```python
from build123d import *

# Parameters (mm, degrees)
SKETCH1_W           = 92
SKETCH1_H           = 80
BOSS_EXTRUDE1_DEPTH = 55
SKETCH2_W           = 78
SKETCH2_H           = 56
CUT_EXTRUDE1_DEPTH  = 50
SKETCH3_W           = 78
SKETCH3_H           = 5
CUT_EXTRUDE2_DEPTH  = 5
FILLET_TOP_R        = 3
FILLET_EDGES_R      = 3
FILLET_BOTTOM_R     = 1
FILLET4_R           = 1
CUT_EXTRUDE4_REACH  = 135.75
SKETCH5_W           = 14
SKETCH5_H           = 14


with BuildPart() as part:
    # Sketch1 → Boss-Extrude1 (new body)
    with BuildSketch(Plane(origin=(0, 0, 0), x_dir=(1, 0, 0), z_dir=(0, 1, 0))):
        with Locations((46, -40)):
            Rectangle(SKETCH1_W, SKETCH1_H)
    extrude(amount=BOSS_EXTRUDE1_DEPTH)

    # Sketch2 → Cut-Extrude1 (cut)
    with BuildSketch(Plane(origin=(0, 55, 0), x_dir=(1, 0, 0), z_dir=(0, 1, 0))):
        with Locations((46, -40)):
            Rectangle(SKETCH2_W, SKETCH2_H)
    extrude(amount=-CUT_EXTRUDE1_DEPTH, mode=Mode.SUBTRACT)

    # Sketch3 → Cut-Extrude2 (cut)
    with BuildSketch(Plane(origin=(0, 55, 0), x_dir=(1, 0, 0), z_dir=(0, 1, 0))):
        with Locations((46, -9.5)):
            Rectangle(SKETCH3_W, SKETCH3_H)
        with Locations((46, -70.5)):
            Rectangle(SKETCH3_W, SKETCH3_H)
    extrude(amount=-CUT_EXTRUDE2_DEPTH, mode=Mode.SUBTRACT)

    # Fillet_top
    fillet_top_edges = [part.edges().sort_by_distance(p)[0] for p in [
        (92, 55, 40),
        (46, 55, 0),
        (0, 55, 40),
        (46, 55, 80),
    ]]
    fillet(fillet_top_edges, radius=FILLET_TOP_R)

    # Fillet_edges
    # the kernel refuses this fillet: 3 mm, written as the material it takes off along each edge
    with BuildSketch(Plane(origin=(3, 52, 77), x_dir=(0, 0, 1), z_dir=(-1, 0, 0))) as fillet_edges_piece_1_section:
        Polygon((0, 0), (FILLET_EDGES_R, 0), (FILLET_EDGES_R, FILLET_EDGES_R), (0, FILLET_EDGES_R), align=None)
    fillet_edges_piece_1 = extrude(amount=FILLET_EDGES_R, mode=Mode.PRIVATE)
    fillet_edges_piece_1 = fillet_edges_piece_1 - Plane(origin=(3, 52, 77), x_dir=(0, -0.7071067811865475, -0.7071067811865475), z_dir=(-1, 0, 0)) * Sphere(FILLET_EDGES_R, mode=Mode.PRIVATE)
    add(fillet_edges_piece_1, mode=Mode.SUBTRACT)
    with BuildSketch(Plane(origin=(3, 52, 3), x_dir=(-1, 0, 0), z_dir=(0, 0, -1))) as fillet_edges_piece_2_section:
        Polygon((0, 0), (FILLET_EDGES_R, 0), (FILLET_EDGES_R, FILLET_EDGES_R), (0, FILLET_EDGES_R), align=None)
    fillet_edges_piece_2 = extrude(amount=FILLET_EDGES_R, mode=Mode.PRIVATE)
    fillet_edges_piece_2 = fillet_edges_piece_2 - Plane(origin=(3, 52, 3), x_dir=(0.7071067811865475, -0.7071067811865475, 0), z_dir=(0, 0, -1)) * Sphere(FILLET_EDGES_R, mode=Mode.PRIVATE)
    add(fillet_edges_piece_2, mode=Mode.SUBTRACT)
    with BuildSketch(Plane(origin=(89, 52, 77), x_dir=(0, 0, 1), z_dir=(1, 0, 0))) as fillet_edges_piece_3_section:
        Polygon((0, 0), (FILLET_EDGES_R, 0), (FILLET_EDGES_R, -FILLET_EDGES_R), (0, -FILLET_EDGES_R), align=None)
    fillet_edges_piece_3 = extrude(amount=FILLET_EDGES_R, mode=Mode.PRIVATE)
    fillet_edges_piece_3 = fillet_edges_piece_3 - Plane(origin=(89, 52, 77), x_dir=(0, -0.7071067811865475, -0.7071067811865475), z_dir=(1, 0, 0)) * Sphere(FILLET_EDGES_R, mode=Mode.PRIVATE)
    add(fillet_edges_piece_3, mode=Mode.SUBTRACT)
    with BuildSketch(Plane(origin=(89, 52, 3), x_dir=(1, 0, 0), z_dir=(0, 0, -1))) as fillet_edges_piece_4_section:
        Polygon((0, 0), (FILLET_EDGES_R, 0), (FILLET_EDGES_R, -FILLET_EDGES_R), (0, -FILLET_EDGES_R), align=None)
    fillet_edges_piece_4 = extrude(amount=FILLET_EDGES_R, mode=Mode.PRIVATE)
    fillet_edges_piece_4 = fillet_edges_piece_4 - Plane(origin=(89, 52, 3), x_dir=(-0.7071067811865475, -0.7071067811865475, 0), z_dir=(0, 0, -1)) * Sphere(FILLET_EDGES_R, mode=Mode.PRIVATE)
    add(fillet_edges_piece_4, mode=Mode.SUBTRACT)
    with BuildSketch(Plane(origin=(92, -7.5, 0), x_dir=(-1, 0, 0), z_dir=(0, 1, 0)), Plane(origin=(92, -7.5, 80), x_dir=(0, 0, -1), z_dir=(0, 1, 0))) as fillet_edges_piece_5:
        with BuildLine():
            CenterArc((FILLET_EDGES_R, FILLET_EDGES_R), FILLET_EDGES_R, 180, 90)
            Line((0, FILLET_EDGES_R), (0, 0))
            Line((0, 0), (FILLET_EDGES_R, 0))
        make_face()
    extrude(amount=59.5, mode=Mode.SUBTRACT)
    with BuildSketch(Plane(origin=(0, -7.5, 80), x_dir=(0, 0, -1), z_dir=(0, 1, 0)), Plane(origin=(0, -7.5, 0), x_dir=(1, 0, 0), z_dir=(0, 1, 0))) as fillet_edges_piece_6:
        with BuildLine():
            CenterArc((FILLET_EDGES_R, -FILLET_EDGES_R), FILLET_EDGES_R, 90, 90)
            Line((0, -FILLET_EDGES_R), (0, 0))
            Line((0, 0), (FILLET_EDGES_R, 0))
        make_face()
    extrude(amount=59.5, mode=Mode.SUBTRACT)

    # Fillet_bottom
    fillet_bottom_edges = [part.edges().sort_by_distance(p)[0] for p in [
        (0, 0, 40),
        (46, 0, 0),
        (92, 0, 40),
        (46, 0, 80),
        (0.878679656, 0, 79.121320344),
        (91.121320344, 0, 79.121320344),
        (91.121320344, 0, 0.878679656),
        (0.878679656, 0, 0.878679656),
    ]]
    fillet(fillet_bottom_edges, radius=FILLET_BOTTOM_R)

    # Fillet4
    fillet4_edges = [part.edges().sort_by_distance(p)[0] for p in [
        (7, 27.5, 68),
        (7, 27.5, 12),
        (85, 27.5, 12),
        (85, 27.5, 68),
        (46, 50, 12),
        (7, 50, 9.5),
        (46, 50, 7),
        (85, 50, 9.5),
        (46, 50, 68),
        (85, 50, 70.5),
        (46, 50, 73),
        (7, 50, 70.5),
    ]]
    fillet(fillet4_edges, radius=FILLET4_R)

    # Sketch5 → Cut-Extrude4 (cut, up to next)
    with BuildSketch(Plane.ZY, mode=Mode.PRIVATE) as cut_extrude4_sk1:
        with Locations((28, 15.5)):
            Rectangle(SKETCH5_W, SKETCH5_H)
    cut_extrude4_tool1 = extrude(cut_extrude4_sk1.sketch, amount=-CUT_EXTRUDE4_REACH, mode=Mode.PRIVATE) & part.part
    add(cut_extrude4_tool1.solids().sort_by_distance((0, 15.5, 28))[0], mode=Mode.SUBTRACT)


solid = part.part
```
Can you work these out from the model? Positions are in its coordinate system, mm. A direction names the side the tool comes from. Coordinates: 2 decimals unless noted, no trailing zeros. Order: outer loops, then holes, each group sorted by start corner. A loop starts at its lowest first (then second) coordinate and runs counter-clockwise, first axis right, second up.
1. Thinking about a two-plate mould opening in Y: for faces 1 (the face through (45, 50, 70)), 2 (the face through (3, 15, 35)), 3 (the face through (45, 53, 73)), which applies, +Y half, -Y half, draft (parallel to the pull), parting line (faces both ways), or undercut?
2. I need wall thicknesses on line 1 (Z direction, x = 10, y = 39); line 2 (X direction, y = 50, z = 30); line 3 (Y direction, x = 30, z = 40). Which ranges of each line are inside material? Lowest first, please.
3. If we section it at A-A (z = 30): Please give me the cut outline in (x, y), then the cut area to 3 significant figures.
4. For faces 4 (the face through (45, 5, 40)), 5 (the face through (3, 8.5, 28)), 6 (the face through (45, 26, 80)), which set-ups out of +Z, -Z, +X, -X, +Y, -Y let a thin tool reach every point of the face, with its end or its side?
5. I'm going to push flat-ended pins straight in: pin 1 (2.5 mm diameter, centred on x = 36.5, z = 70, fed in from +Y); pin 2 (1.2 mm diameter, centred on x = 35.5, y = 53.5, fed in from -Z). Where does each tip first touch, or does it pass through?
6. If we section it at D-D (z = 40.5): Please give me the cut outline in (x, y).
7. If we section it at C-C (x = 56.5): Please give me the cut outline in (y, z).
8. If we section it at B-B (y = 42.5): Please give me the cut outline in (x, z), then the cut area to 3 significant figures.
Entries:
1. face 1: +Y half
1. face 2: undercut
1. face 3: draft
2. line 1: z = 0 to 12, 68 to 80
2. line 2: x = 0 to 7, 85 to 92
2. line 3: y = 0 to 5
3. outline: (0, 1) arc R1 ccw to (1, 0) - (91, 0) arc R1 ccw to (92, 1) - (92, 52) arc R3 ccw to (89, 55) - (85, 55) - (85, 5) - (7, 5) - (7, 8.5) - (0, 8.5) - close; (0, 22.5) - (7, 22.5) - (7, 55) - (3, 55) arc R3 ccw to (0, 52) - close
3. area: 1,060 mm2
4. face 4: +Y
4. face 5: -X
4. face 6: +Z, +X, -X, +Y, -Y
5. pin 1: stops at y = 50
5. pin 2: stops at z = 0.14
6. outline: (0, 1) arc R1 ccw to (1, 0) - (91, 0) arc R1 ccw to (92, 1) - (92, 52) arc R3 ccw to (89, 55) - (85, 55) - (85, 5) - (7, 5) - (7, 55) - (3, 55) arc R3 ccw to (0, 52) - close
7. outline: (0, 1) arc R1 ccw to (1, 0) - (52, 0) arc R3 ccw to (55, 3) - (55, 7) - (51, 7) arc R1 cw to (50, 8) - (50, 11) arc R1 ccw to (49, 12) - (5, 12) - (5, 68) - (49, 68) arc R1 ccw to (50, 69) - (50, 72) arc R1 cw to (51, 73) - (55, 73) - (55, 77) arc R3 ccw to (52, 80) - (1, 80) arc R1 ccw to (0, 79) - close
8. outline: (0, 3) arc R3 ccw to (3, 0) - (89, 0) arc R3 ccw to (92, 3) - (92, 77) arc R3 ccw to (89, 80) - (3, 80) arc R3 ccw to (0, 77) - close; hole (7, 13) arc R1 ccw to (8, 12) - (84, 12) arc R1 ccw to (85, 13) - (85, 67) arc R1 ccw to (84, 68) - (8, 68) arc R1 ccw to (7, 67) - close
8. area: 2,990 mm2
